Print and shaded views of the part. All mm, measured from the part's lowest x, y and z. A direction names the side the tool comes from. Round coordinates to 2 decimals unless told otherwise and drop trailing zeros. Loops run counter-clockwise (first coordinate to the right, second up) from the corner with the lowest first, then second, coordinate; pieces in that order, holes last. Notation, with made-up numbers: (38, 11) -> (93, 11) arc R25 ccw to (93, 47) -> close; hole circle Ø5 at (-33.75, 14). An arc over 180 degrees is marked (long way). Answer as CSV lines item,"result".
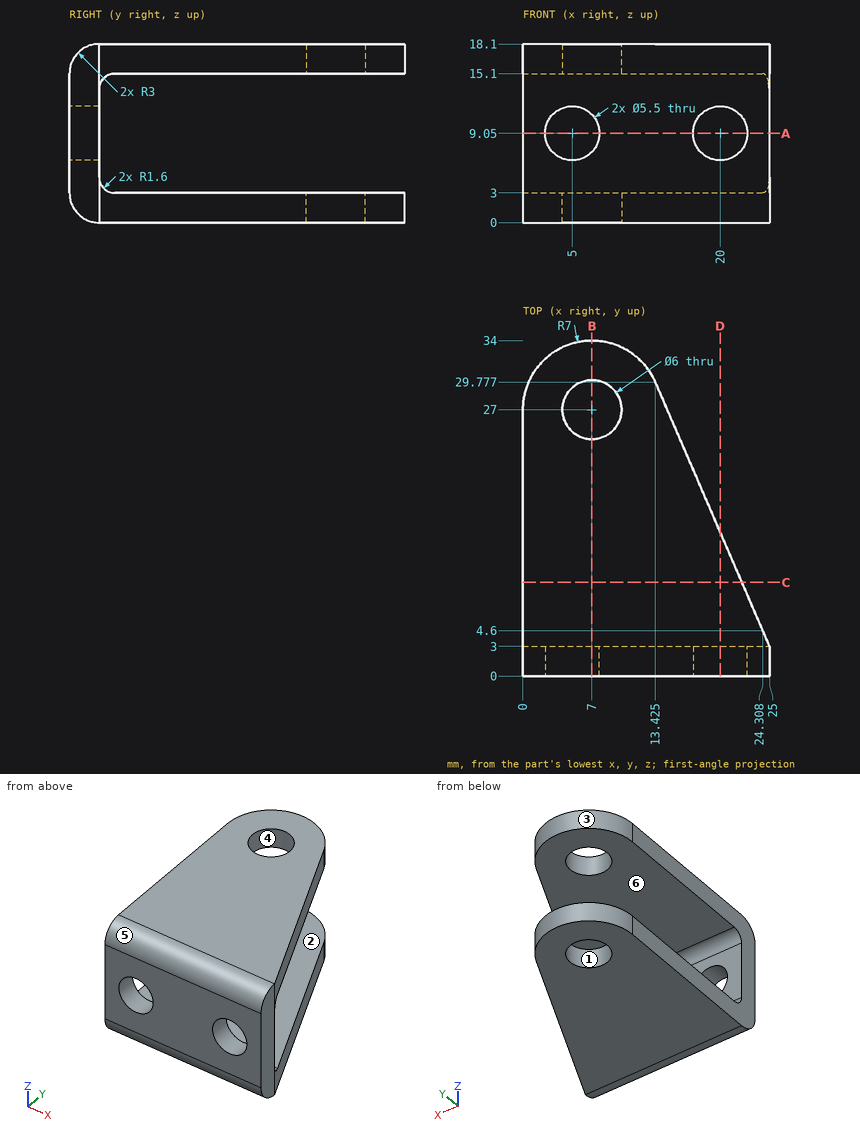
Q1. Drill centre lines: line 1 along X through (y, z) = (2.2, 9.05); line 2 along Z through (x, y) = (12.75, 7); line 3 along Z through (x, y) = (21, 2). Where is each one in solid material? Low to high.
Geometry results:
line 1,"0 to 2.25, 7.75 to 17.25, 22.75 to 25"
line 2,"0 to 3, 15.1 to 18.1"
line 3,"0.17 to 6.49, 11.61 to 17.93"
Q2. Saw through at A-A, the plane z = 9.05. Write the cut outline in (x, y).
Geometry results:
outline,"(0, 0) -> (2.25, 0) -> (2.25, 3) -> (0, 3) -> close; (7.75, 0) -> (17.25, 0) -> (17.25, 3) -> (7.75, 3) -> close; (22.75, 0) -> (25, 0) -> (25, 3) -> (22.75, 3) -> close"
Q3. Saw through at D-D, the plane x = 20. Write the cut outline in (y, z).
Geometry results:
outline,"(0, 3) arc R3 ccw to (3, 0) -> (14.57, 0) -> (14.57, 3) -> (4.6, 3) arc R1.6 cw to (3, 4.6) -> (3, 6.3) -> (0, 6.3) -> close; (0, 11.8) -> (3, 11.8) -> (3, 13.5) arc R1.6 cw to (4.6, 15.1) -> (14.57, 15.1) -> (14.57, 18.1) -> (3, 18.1) arc R3 ccw to (0, 15.1) -> close"
Q4. Saw through at B-B, the plane x = 7. Write the cut outline in (y, z).
Geometry results:
outline,"(0, 3) arc R3 ccw to (3, 0) -> (24, 0) -> (24, 3) -> (4.6, 3) arc R1.6 cw to (3, 4.6) -> (3, 7.16) -> (0, 7.16) -> close; (0, 10.94) -> (3, 10.94) -> (3, 13.5) arc R1.6 cw to (4.6, 15.1) -> (24, 15.1) -> (24, 18.1) -> (3, 18.1) arc R3 ccw to (0, 15.1) -> close; (30, 0) -> (34, 0) -> (34, 3) -> (30, 3) -> close; (30, 15.1) -> (34, 15.1) -> (34, 18.1) -> (30, 18.1) -> close"
Q5. Saw through at C-C, the plane y = 9.5. Write the cut outline in (x, z).
Geometry results:
outline,"(0, 0) -> (22.19, 0) -> (22.19, 3) -> (0, 3) -> close; (0, 15.1) -> (22.19, 15.1) -> (22.19, 18.1) -> (0, 18.1) -> close"
Q6. Which spindle directions (+Z, -Z, +X, -X, +Y, -Y) get a long thin tool onto all of the face, cutting with end or side? Do the marked faces 5 and 6. Say none if no direction does.
Geometry results:
face 5,"+Z, +X, -X, -Y"
face 6,"+X, -X, +Y"
Q7. Drop a flat-ended pin along its axis: P1, Ø8, axis at x = 17, z = 9.5, coming from the +Y side. Give the stop position or say it passes through.
Geometry results:
P1,"y = 3"
Q8. Two-plate mould, pull along X, no slides. Class the marked faces 1, 2, 3 and 4: pulls with the +X half, pulls with the -X half, needs draft (parallel to the pull), parting line crosses it, or undercut.
Geometry results:
face 1,"undercut"
face 2,"needs draft"
face 3,"parting line crosses it"
face 4,"undercut"
